```python
from build123d import *

# Parameters (mm, degrees)
BASE_FLANGE1_DEPTH             = 30
EDGE_FLANGE3_STRIP_W           = 9.4732
EDGE_FLANGE3_STRIP_H           = 2
EDGE_FLANGE3_STRIP_CUT_DEPTH   = 23.982438423
EDGE_FLANGE3_STRIP_2_W         = 9.4732
EDGE_FLANGE3_STRIP_2_H         = 2
EDGE_FLANGE3_STRIP_CUT_2_DEPTH = 23.982438423
EDGE_FLANGE3_STRIP_3_W         = 9.4732
EDGE_FLANGE3_STRIP_3_H         = 2
EDGE_FLANGE3_STRIP_CUT_3_DEPTH = 22.356175112
EDGE_FLANGE3_STRIP_4_W         = 9.4732
EDGE_FLANGE3_STRIP_4_H         = 2
EDGE_FLANGE3_STRIP_CUT_4_DEPTH = 22.356175112
EDGE_FLANGE3_STRIP_5_W         = 9.4732
EDGE_FLANGE3_STRIP_5_H         = 2
EDGE_FLANGE3_STRIP_CUT_5_DEPTH = 77.034991311
EDGE_FLANGE3_STRIP_6_W         = 9.4732
EDGE_FLANGE3_STRIP_6_H         = 2
EDGE_FLANGE3_STRIP_CUT_6_DEPTH = 77.034991311
EDGE_FLANGE3_DEPTH             = 23.982438423
EDGE_FLANGE3_BEND_DEPTH        = 23.982438423
EDGE_FLANGE3_BEND_2_DEPTH      = 22.356175112
EDGE_FLANGE3_BEND_3_DEPTH      = 22.356175112
EDGE_FLANGE3_BEND_4_DEPTH      = 77.034991311
EDGE_FLANGE3_BEND_5_DEPTH      = 77.034991311
CUT_EXTRUDE1_REACH             = 114.784
SKETCH35_R                     = 1.75
SKETCH35_R_2                   = 2


# Sheet-metal steps are written as plain solids
with BuildPart() as part:
    # Sketch1 → Base-Flange1 (new body)
    with BuildSketch(Plane.XY):
        with BuildLine():
            Line((0, 0), (23.982438423, 0))
            ThreePointArc((23.982438423, 0), (24.316990043, 0.080357077), (24.578547934, 0.3038957))
            Line((24.578547934, 0.3038957), (69.831564503, 62.646131606))
            ThreePointArc((69.831564503, 62.646131606), (69.891697915, 63.413387526), (69.235454992, 63.815435906))
            Line((69.235454992, 63.815435906), (46.87927988, 63.815435906))
            Line((46.87927988, 63.815435906), (46.87927988, 65.815435906))
            Line((46.87927988, 65.815435906), (69.235454992, 65.815435906))
            ThreePointArc((69.235454992, 65.815435906), (71.673514159, 64.321754671), (71.450107838, 61.471262477))
            Line((71.450107838, 61.471262477), (26.19709127, -0.870973429))
            ThreePointArc((26.19709127, -0.870973429), (25.225357188, -1.701459167), (23.982438423, -2))
            Line((23.982438423, -2), (0, -2))
            Line((0, -2), (0, 0))
        make_face()
    extrude(amount=BASE_FLANGE1_DEPTH)

    # Edge-Flange3 strip (across the edge) → Edge-Flange3 strip cut (cut)
    with BuildSketch(Plane(origin=(0, -2, 0), x_dir=(0, 0, 1), z_dir=(1, 0, 0))):
        with Locations((-2, -1)):
            Rectangle(EDGE_FLANGE3_STRIP_W, EDGE_FLANGE3_STRIP_H)
    extrude(amount=EDGE_FLANGE3_STRIP_CUT_DEPTH, mode=Mode.SUBTRACT)

    # Edge-Flange3 strip 2 (across the edge) → Edge-Flange3 strip cut 2 (cut)
    with BuildSketch(Plane(origin=(23.982438423, -2, 30), x_dir=(0, 0, -1), z_dir=(-1, 0, 0))):
        with Locations((-2, -1)):
            Rectangle(EDGE_FLANGE3_STRIP_2_W, EDGE_FLANGE3_STRIP_2_H)
    extrude(amount=EDGE_FLANGE3_STRIP_CUT_2_DEPTH, mode=Mode.SUBTRACT)

    # Edge-Flange3 strip 3 (across the edge) → Edge-Flange3 strip cut 3 (cut)
    with BuildSketch(Plane(origin=(46.87927988, 65.815435906, 30), x_dir=(0, 0, -1), z_dir=(1, 0, 0))):
        with Locations((-2, -1)):
            Rectangle(EDGE_FLANGE3_STRIP_3_W, EDGE_FLANGE3_STRIP_3_H)
    extrude(amount=EDGE_FLANGE3_STRIP_CUT_3_DEPTH, mode=Mode.SUBTRACT)

    # Edge-Flange3 strip 4 (across the edge) → Edge-Flange3 strip cut 4 (cut)
    with BuildSketch(Plane(origin=(69.235454992, 65.815435906, 0), x_dir=(0, 0, 1), z_dir=(-1, 0, 0))):
        with Locations((-2, -1)):
            Rectangle(EDGE_FLANGE3_STRIP_4_W, EDGE_FLANGE3_STRIP_4_H)
    extrude(amount=EDGE_FLANGE3_STRIP_CUT_4_DEPTH, mode=Mode.SUBTRACT)

    # Edge-Flange3 strip 5 (across the edge) → Edge-Flange3 strip cut 5 (cut)
    with BuildSketch(Plane(origin=(26.19709127, -0.870973429, 0), x_dir=(0, 0, 1), z_dir=(0.5874345644557342, 0.8092716679105367, 0))):
        with Locations((-2, -1)):
            Rectangle(EDGE_FLANGE3_STRIP_5_W, EDGE_FLANGE3_STRIP_5_H)
    extrude(amount=EDGE_FLANGE3_STRIP_CUT_5_DEPTH, mode=Mode.SUBTRACT)

    # Edge-Flange3 strip 6 (across the edge) → Edge-Flange3 strip cut 6 (cut)
    with BuildSketch(Plane(origin=(71.450107838, 61.471262477, 30), x_dir=(0, 0, -1), z_dir=(-0.5874345644557342, -0.8092716679105367, 0))):
        with Locations((-2, -1)):
            Rectangle(EDGE_FLANGE3_STRIP_6_W, EDGE_FLANGE3_STRIP_6_H)
    extrude(amount=EDGE_FLANGE3_STRIP_CUT_6_DEPTH, mode=Mode.SUBTRACT)

    # Edge-Flange3 section (across the edge) → Edge-Flange3 (add)
    with BuildSketch(Plane(origin=(0, -2, 0), x_dir=(0, 0, 1), z_dir=(1, 0, 0))):
        with BuildLine():
            Line((0, 0.7366), (0, 8))
            Line((0, 8), (2, 8))
            Line((2, 8), (2, 0.7366))
            ThreePointArc((2, 0.7366), (2.215745145, 0.215745145), (2.7366, 0))
            Line((2.7366, 0), (2.7366, -2))
            ThreePointArc((2.7366, -2), (0.801531583, -1.198468417), (0, 0.7366))
        make_face()
    extrude(amount=EDGE_FLANGE3_DEPTH)

    # Edge-Flange3 section 2 (across the edge) → Edge-Flange3 bend (add)
    with BuildSketch(Plane(origin=(23.982438423, -2, 30), x_dir=(0, 0, -1), z_dir=(-1, 0, 0))):
        with BuildLine():
            Line((0, 0.7366), (0, 8))
            Line((0, 8), (2, 8))
            Line((2, 8), (2, 0.7366))
            ThreePointArc((2, 0.7366), (2.215745145, 0.215745145), (2.7366, 0))
            Line((2.7366, 0), (2.7366, -2))
            ThreePointArc((2.7366, -2), (0.801531583, -1.198468417), (0, 0.7366))
        make_face()
    extrude(amount=EDGE_FLANGE3_BEND_DEPTH)

    # Edge-Flange3 section 3 (across the edge) → Edge-Flange3 bend 2 (add)
    with BuildSketch(Plane(origin=(46.87927988, 65.815435906, 30), x_dir=(0, 0, -1), z_dir=(1, 0, 0))):
        with BuildLine():
            Line((0, 0.7366), (0, 8))
            Line((0, 8), (2, 8))
            Line((2, 8), (2, 0.7366))
            ThreePointArc((2, 0.7366), (2.215745145, 0.215745145), (2.7366, 0))
            Line((2.7366, 0), (2.7366, -2))
            ThreePointArc((2.7366, -2), (0.801531583, -1.198468417), (0, 0.7366))
        make_face()
    extrude(amount=EDGE_FLANGE3_BEND_2_DEPTH)

    # Edge-Flange3 section 4 (across the edge) → Edge-Flange3 bend 3 (add)
    with BuildSketch(Plane(origin=(69.235454992, 65.815435906, 0), x_dir=(0, 0, 1), z_dir=(-1, 0, 0))):
        with BuildLine():
            Line((0, 0.7366), (0, 8))
            Line((0, 8), (2, 8))
            Line((2, 8), (2, 0.7366))
            ThreePointArc((2, 0.7366), (2.215745145, 0.215745145), (2.7366, 0))
            Line((2.7366, 0), (2.7366, -2))
            ThreePointArc((2.7366, -2), (0.801531583, -1.198468417), (0, 0.7366))
        make_face()
    extrude(amount=EDGE_FLANGE3_BEND_3_DEPTH)

    # Edge-Flange3 section 5 (across the edge) → Edge-Flange3 bend 4 (add)
    with BuildSketch(Plane(origin=(26.19709127, -0.870973429, 0), x_dir=(0, 0, 1), z_dir=(0.5874345644557342, 0.8092716679105367, 0))):
        with BuildLine():
            Line((0, 0.7366), (0, 8))
            Line((0, 8), (2, 8))
            Line((2, 8), (2, 0.7366))
            ThreePointArc((2, 0.7366), (2.215745145, 0.215745145), (2.7366, 0))
            Line((2.7366, 0), (2.7366, -2))
            ThreePointArc((2.7366, -2), (0.801531583, -1.198468417), (0, 0.7366))
        make_face()
    extrude(amount=EDGE_FLANGE3_BEND_4_DEPTH)

    # Edge-Flange3 section 6 (across the edge) → Edge-Flange3 bend 5 (add)
    with BuildSketch(Plane(origin=(71.450107838, 61.471262477, 30), x_dir=(0, 0, -1), z_dir=(-0.5874345644557342, -0.8092716679105367, 0))):
        with BuildLine():
            Line((0, 0.7366), (0, 8))
            Line((0, 8), (2, 8))
            Line((2, 8), (2, 0.7366))
            ThreePointArc((2, 0.7366), (2.215745145, 0.215745145), (2.7366, 0))
            Line((2.7366, 0), (2.7366, -2))
            ThreePointArc((2.7366, -2), (0.801531583, -1.198468417), (0, 0.7366))
        make_face()
    extrude(amount=EDGE_FLANGE3_BEND_5_DEPTH)

    # Sketch35 → Cut-Extrude1 (cut, up to next)
    with BuildSketch(Plane(origin=(0, 65.815435906, 0), x_dir=(1, 0, 0), z_dir=(0, 1, 0)), mode=Mode.PRIVATE) as cut_extrude1_sk1:
        with Locations(Location((6.128769165, -6.128769165, 0), (0, 0, 270))):
            Circle(SKETCH35_R)
    cut_extrude1_tool1 = extrude(cut_extrude1_sk1.sketch, amount=-CUT_EXTRUDE1_REACH, mode=Mode.PRIVATE) & part.part
    # Sketch35 → Cut-Extrude1 (cut, up to next)
    with BuildSketch(Plane(origin=(0, 65.815435906, 0), x_dir=(1, 0, 0), z_dir=(0, 1, 0)), mode=Mode.PRIVATE) as cut_extrude1_sk2:
        with Locations(Location((18.374243868, -6.128769165, 0), (0, 0, 270))):
            Circle(SKETCH35_R)
    cut_extrude1_tool2 = extrude(cut_extrude1_sk2.sketch, amount=-CUT_EXTRUDE1_REACH, mode=Mode.PRIVATE) & part.part
    # Sketch35 → Cut-Extrude1 (cut, up to next)
    with BuildSketch(Plane(origin=(0, 65.815435906, 0), x_dir=(1, 0, 0), z_dir=(0, 1, 0)), mode=Mode.PRIVATE) as cut_extrude1_sk3:
        with Locations(Location((6.128769165, -23.871230835, 0), (0, 0, 270))):
            Circle(SKETCH35_R)
    cut_extrude1_tool3 = extrude(cut_extrude1_sk3.sketch, amount=-CUT_EXTRUDE1_REACH, mode=Mode.PRIVATE) & part.part
    # Sketch35 → Cut-Extrude1 (cut, up to next)
    with BuildSketch(Plane(origin=(0, 65.815435906, 0), x_dir=(1, 0, 0), z_dir=(0, 1, 0)), mode=Mode.PRIVATE) as cut_extrude1_sk4:
        with Locations(Location((18.374243868, -23.871230835, 0), (0, 0, 270))):
            Circle(SKETCH35_R)
    cut_extrude1_tool4 = extrude(cut_extrude1_sk4.sketch, amount=-CUT_EXTRUDE1_REACH, mode=Mode.PRIVATE) & part.part
    # Sketch35 → Cut-Extrude1 (cut, up to next)
    with BuildSketch(Plane(origin=(0, 65.815435906, 0), x_dir=(1, 0, 0), z_dir=(0, 1, 0)), mode=Mode.PRIVATE) as cut_extrude1_sk5:
        with Locations(Location((58.057367436, -15, 0), (0, 0, 270))):
            Circle(SKETCH35_R_2)
    cut_extrude1_tool5 = extrude(cut_extrude1_sk5.sketch, amount=-CUT_EXTRUDE1_REACH, mode=Mode.PRIVATE) & part.part
    add(cut_extrude1_tool1.solids().sort_by_distance((6.128769, 65.815436, 6.128769))[0], mode=Mode.SUBTRACT)
    add(cut_extrude1_tool2.solids().sort_by_distance((18.374244, 65.815436, 6.128769))[0], mode=Mode.SUBTRACT)
    add(cut_extrude1_tool3.solids().sort_by_distance((6.128769, 65.815436, 23.871231))[0], mode=Mode.SUBTRACT)
    add(cut_extrude1_tool4.solids().sort_by_distance((18.374244, 65.815436, 23.871231))[0], mode=Mode.SUBTRACT)
    add(cut_extrude1_tool5.solids().sort_by_distance((58.057367, 65.815436, 15))[0], mode=Mode.SUBTRACT)


solid = part.part
```
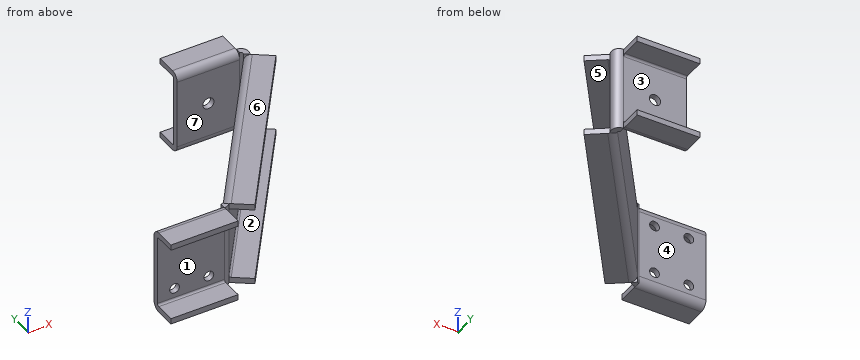
Work out the finished part from the listing and answer in its coordinate system (mm). Face numbers are marked on the shaded views. A direction names the side the tool comes from. Give positions to 0.01 mm unless a question says otherwise; leave off trailing zeros. Write each loop counter-clockwise with the first axis right and the second up, starting at its lowest first coordinate (ties: lowest second). Pieces come first, ordered by that corner, then holes.
(1) The mould has two halves that part along Z. Classify the marked faces 5, 6 and 7: pulls with the +Z half, pulls with the -Z half, needs draft (parallel to the pull), parting line crosses it, or undercut.
Final values:
face 5: undercut
face 6: pulls with the +Z half
face 7: needs draft
(2) Flat-ended cylindrical pins translate along their axes: pin 1 Ø2 at (x, z) = (15, 12) entering from +Y; pin 2 Ø1.4 at (y, z) = (68.5, 1.5) entering from +X; pin 3 Ø8 at (x, z) = (16.5, 7.5) entering from -Y. Find the tip coordinate at first contact, or state that the pin passes through.
Final values:
pin 1: stops at y = 0
pin 2: stops at x = 69.24
pin 3: stops at y = -2
(3) The part is cut by section A-A on z = 15. Write down the section's boundary in (x, y).
Final values:
outline: (0, -2) - (23.98, -2) arc R2.74 ccw to (26.2, -0.87) - (71.45, 61.47) arc R2.74 ccw to (69.24, 65.82) - (60.06, 65.82) - (60.06, 63.82) - (69.24, 63.82) arc R0.74 cw to (69.83, 62.65) - (24.58, 0.3) arc R0.74 cw to (23.98, 0) - (0, 0) - close; (46.88, 63.82) - (56.06, 63.82) - (56.06, 65.82) - (46.88, 65.82) - close
(4) Which of the six approach directions +Z, -Z, +X, -X, +Y, -Y give full straight-line access (tool end or side, diameter ignored) to the marked faces 1, 2, 3 and 4?
Final values:
face 1: +X, -X, -Y
face 2: +X, -Y
face 3: +X, -X, +Y
face 4: +Z, -Z, -X, +Y
(5) Straight lines are drawn through the part: line 1 (Z direction, x = 68.5, y = 69.5); line 2 (Y direction, x = 12, z = 4.5); line 3 (X direction, y = 64.75, z = 15). For each, find the intervals that lie inside material, in ascending order.
Final values:
line 1: z = 0 to 2, 28 to 30
line 2: y = -2 to 0
line 3: x = 46.88 to 56.06, 60.06 to 71.4
